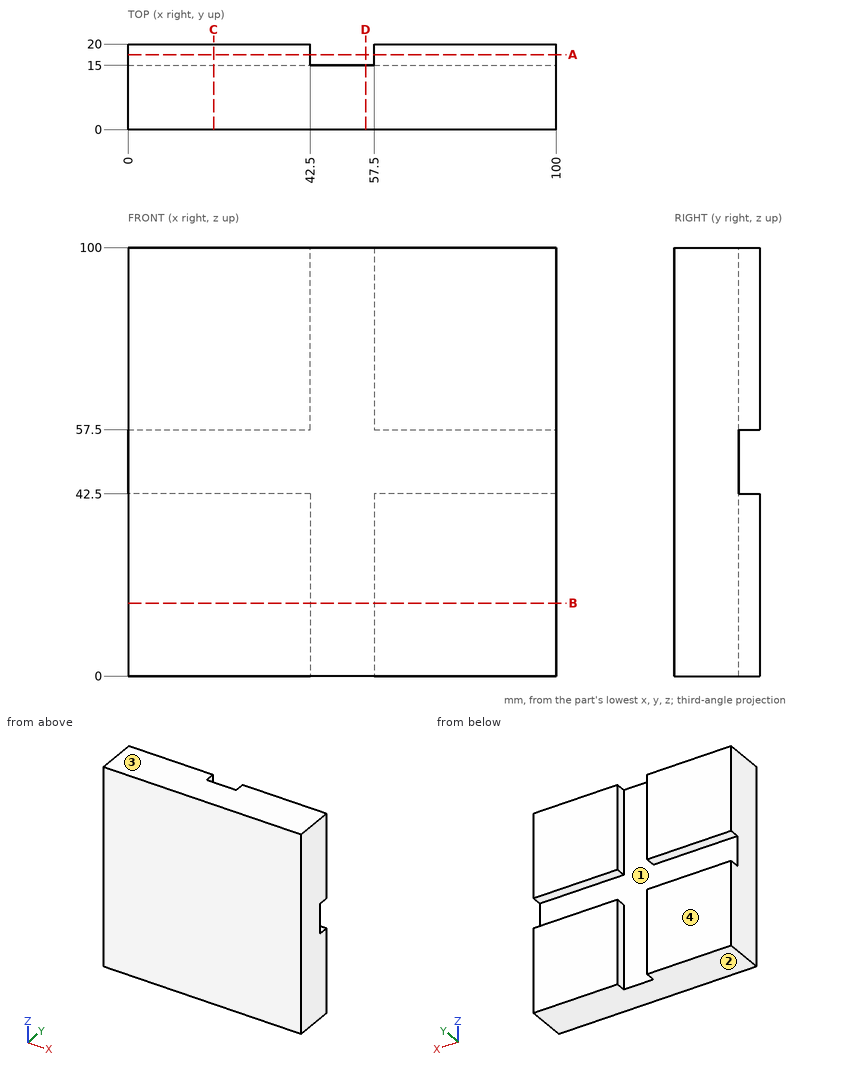
Geometry check sheet. Reference: drawing and pictorial views, mm from the part's lowest x, y, z. Round coordinates to 2 decimals unless told otherwise and drop trailing zeros. Write each loop counter-clockwise with the first axis right and the second up, starting at its lowest first coordinate (ties: lowest second). Pieces come first, ordered by that corner, then holes.
Item 1: Go/stop test with a flat-tipped pin: pin 1 Ø10 at (y, z) = (4.5, 67.5) entering from -X. Record where the tip stops, or that it passes through.
Determined:
pin 1: stops at x = 0
Item 2: Section check C-C (x = 20). Record the boundary of the cut face in (y, z).
Determined:
outline: (0, 0) - (20, 0) - (20, 42.5) - (15, 42.5) - (15, 57.5) - (20, 57.5) - (20, 100) - (0, 100) - close
Item 3: Section check A-A (y = 17.5). Record the boundary of the cut face in (x, z), plus the area to 4 significant figures.
Determined:
outline: (0, 0) - (42.5, 0) - (42.5, 42.5) - (0, 42.5) - close; (0, 57.5) - (42.5, 57.5) - (42.5, 100) - (0, 100) - close; (57.5, 0) - (100, 0) - (100, 42.5) - (57.5, 42.5) - close; (57.5, 57.5) - (100, 57.5) - (100, 100) - (57.5, 100) - close
area: 7,225 mm2
Item 4: Mould release check, pull along Z, two halves, no side actions. Record for the marked faces 1, 2, 3 and 4: +Z half, -Z half, draft (parallel to the pull), parting line (faces both ways), or undercut.
Determined:
face 1: undercut
face 2: -Z half
face 3: +Z half
face 4: draft
Item 5: Section check D-D (x = 55.5). Record the boundary of the cut face in (y, z).
Determined:
outline: (0, 0) - (15, 0) - (15, 100) - (0, 100) - close
Item 6: Material ranges on line 1 along X through (y, z) = (17.25, 69); line 2 along Y through (x, z) = (43, 59), recorded low to high.
Determined:
line 1: x = 0 to 42.5, 57.5 to 100
line 2: y = 0 to 15
Item 7: Section check B-B (z = 17). Record the boundary of the cut face in (x, y), plus the area to 4 significant figures.
Determined:
outline: (0, 0) - (100, 0) - (100, 20) - (57.5, 20) - (57.5, 15) - (42.5, 15) - (42.5, 20) - (0, 20) - close
area: 1,925 mm2
